Part print with two shaded views. Sizes in mm from the minimum x, y, z corner. A direction names the side the tool comes from. Coordinates: 2 decimals unless noted, no trailing zeros. Loops run counter-clockwise (first coordinate to the right, second up) from the corner with the lowest first, then second, coordinate; pieces in that order, holes last.
(1) Tool access for the marked faces 4, 5, 6 and 7: list every direction of +Z, -Z, +X, -X, +Y, -Y with a clear straight run to the whole face (end or side of a thin tool).
(2) Flat gauge pin, fed straight in: P1, Ø0.9, axis at x = 11.5, y = 1.5, coming from the +Z side. Where does the tip first touch, or does it go through?
(3) Slice it at A-A (z = 14.75). Give the cut face in (x, y).
(4) Two-plate mould, pull along Z, no slides. Class the marked faces 1, 2 and 3: pulls with the +Z half, pulls with the -Z half, needs draft (parallel to the pull), parting line crosses it, or undercut.
(5) Slice it at C-C (x = 15). Give the cut face in (y, z), and give its area (3 significant figures).
(6) Wall check: L1, parallel to X at y = 2.1, z = 7.25; L2, parallel to X at y = 2.6, z = 14.25; L3, parallel to Z at x = 4.25, y = 1.3. Give the ranges that are in metal, low to high.
(7) Slice it at B-B (y = 0.4). Give the cut face in (x, z).
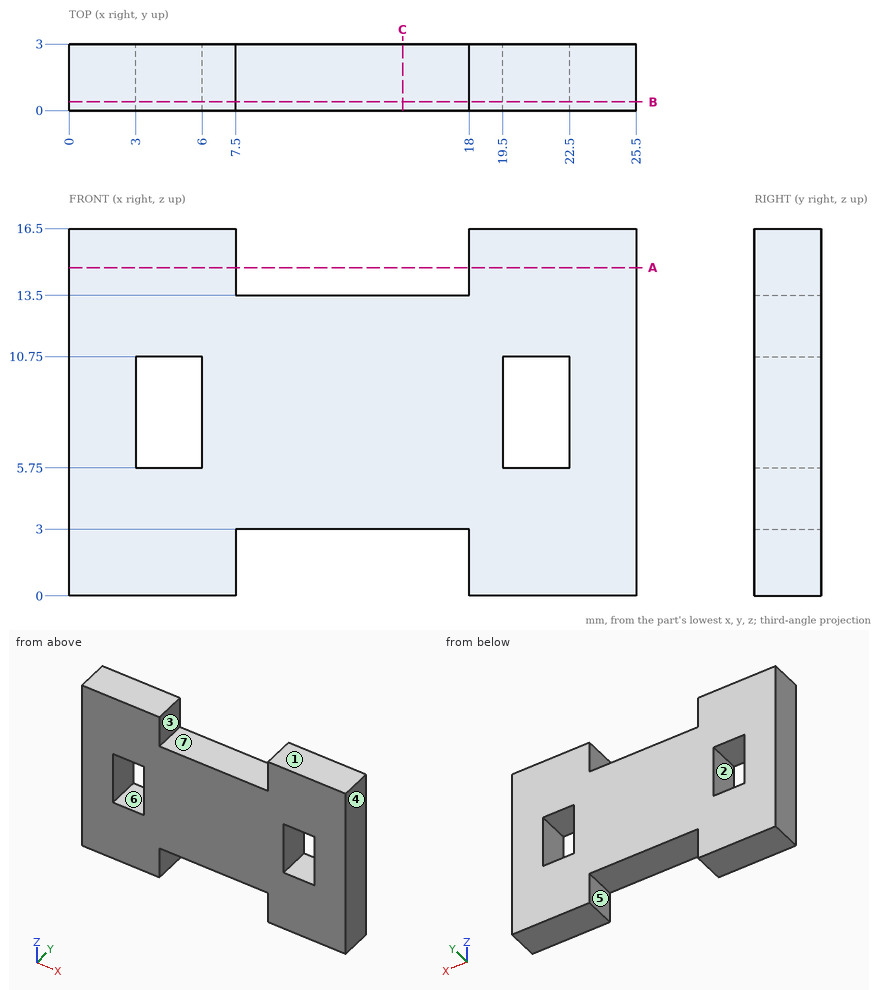
Response values:
1. face 4: +Z, -Z, +X, +Y, -Y
1. face 5: -Z, +Y, -Y
1. face 6: +Y, -Y
1. face 7: +Z, +Y, -Y
2. P1: stops at z = 13.5
3. outline: (0, 0) - (7.5, 0) - (7.5, 3) - (0, 3) - close; (18, 0) - (25.5, 0) - (25.5, 3) - (18, 3) - close
4. face 1: pulls with the +Z half
4. face 2: undercut
4. face 3: needs draft
5. outline: (0, 3) - (3, 3) - (3, 13.5) - (0, 13.5) - close
5. area: 31.5 mm2
6. L1: x = 0 to 3, 6 to 19.5, 22.5 to 25.5
6. L2: x = 0 to 7.5, 18 to 25.5
6. L3: z = 0 to 5.75, 10.75 to 16.5
7. outline: (0, 0) - (7.5, 0) - (7.5, 3) - (18, 3) - (18, 0) - (25.5, 0) - (25.5, 16.5) - (18, 16.5) - (18, 13.5) - (7.5, 13.5) - (7.5, 16.5) - (0, 16.5) - close; hole (3, 5.75) - (6, 5.75) - (6, 10.75) - (3, 10.75) - close; hole (19.5, 5.75) - (22.5, 5.75) - (22.5, 10.75) - (19.5, 10.75) - close
